Check sheet for the modelled part. Datum: model origin and axes. Units: mm. Give positions to 0.01 mm unless a question says otherwise; leave off trailing zeros. Write each loop counter-clockwise with the first axis right and the second up, starting at its lowest first coordinate (ties: lowest second). Pieces come first, ordered by that corner, then holes. Notation, with made-up numbers: M 6.25,35.25 L 22.25,35.25 A24 cw 22.25,69.25 Z; hole C 19.25,-22 d6. An arc over 180 degrees is marked long. Write item = value, one per line. Start each with the question number.
1) Mould release check, pull along Z, two halves, no side actions. Record for faces 1 (the cylindrical face through (-41.288, 0.507, -39.063)), 2 (the flat face through (-52, 0, -30)): released by +Z, released by -Z, zero draft, split by the parting line, or undercut.
2) Scan lines: line 1 along X through (y, z) = (0.8, -28.5); line 2 along X through (y, z) = (0.2, -39.5); line 3 along Z through (x, y) = (-17, 0.5). Record each from-to range of solid material in increasing order. Write a range as [from, to].
3) Go/stop test with a flat-tipped pin: pin 1 (2.5 mm diameter, centred on x = -40.1, z = -39.98, fed in from +Y). Record where the tip stops, or that it passes through.
4) Cross-section at B-B, the plane y = 0.4. Record the cut outline in (x, z).
5) Cross-section at A-A, the plane z = -30. Record the cut outline in (x, y), plus the area to 3 significant figures.
Autodesk Inventor part; units mm, degrees
ref_plane "YZ Plane" through (0, 0, 0) normal (1, 0, 0) x (0, 1, 0)
ref_plane "XZ Plane" through (0, 0, 0) normal (0, 1, 0) x (-1, 0, 0)
ref_plane "XY Plane" through (0, 0, 0) normal (0, 0, 1) x (1, 0, 0)
sketch "Sketch1" plane through (0, 0, 0) normal (0, 1, 0) x (-1, 0, 0)
  line L0 (100, 0) -> (100, -60)
  line L1 (5, -60) -> (5, 0)
  line L2 (100, -60) -> (5, -60)
  line L3 (100, 0) -> (5, 0)
  point P0 (0, 0)
  dimension "d1" = 60
extrude "Extrusion1" add sketch "Sketch1" along normal blind 1
sketch "Sketch3" plane through (0, 1, 0) normal (0, 1, 0) x (1, 0, 0)
  point P0 (0, 0)
sketch "Sketch4" plane through (0, 1, 0) normal (0, 1, 0) x (1, 0, 0)
  point P0 (0, 0)
sketch "Sketch5" plane through (0, 1, 0) normal (0, 1, 0) x (1, 0, 0)
  circle A0 centre (-40.098, 20.0247) radius 1.5
  circle A1 centre (-40.098, 39.9753) radius 1.5
  circle A2 centre (-15.013, 30) radius 6.5
  point P0 (0, 0)
  dimension "d9" = 3
  dimension "d10" = 3
  dimension "d11" = 13
extrude "Extrusion3" cut sketch "Sketch5" against normal blind 1
properties part number "striking"
Reply:
q1.face_1 = undercut
q1.face_2 = zero draft
q2.line_1 = [-100, -21.34], [-8.69, -5]
q2.line_2 = [-100, -41.52], [-38.68, -5]
q2.line_3 = [-60, -36.19], [-23.81, 0]
q3.pin_1 = through
q4.outline = M -100,-60 L -5,-60 L -5,0 L -100,0 Z; hole C -40.1,-39.98 d3; hole C -40.1,-20.02 d3; hole C -15.01,-30 d13
q5.outline = M -100,0 L -21.51,0 L -21.51,1 L -100,1 Z; M -8.51,0 L -5,0 L -5,1 L -8.51,1 Z
q5.area = 82.0 mm2
